```python
from build123d import *

# Parameters (mm, degrees)
BOSS_EXTRUDE1_DEPTH = 4.5
CUT_EXTRUDE1_DEPTH  = 24.873773295
FILLET1_R           = 10
FILLET2_R           = 1


with BuildPart() as part:
    # Sketch1 → Boss-Extrude1 (new body)
    with BuildSketch(Plane.XY):
        with BuildLine():
            ThreePointArc((1.715540677, -1.028066236), (0, 2), (-1.715540677, -1.028066236))
            ThreePointArc((-1.715540677, -1.028066236), (-12.4000088, -2.631992998), (-22.452233946, -6.592196245))
            ThreePointArc((-22.452233946, -6.592196245), (-18.208029962, 2.594911639), (-8.117877526, 3.372756458))
            ThreePointArc((-8.117877526, 3.372756458), (0, 4), (8.117877526, 3.372756458))
            ThreePointArc((8.117877526, 3.372756458), (18.208029962, 2.594911639), (22.452233946, -6.592196245))
            ThreePointArc((22.452233946, -6.592196245), (12.4000088, -2.631992998), (1.715540677, -1.028066236))
        make_face()
    extrude(amount=BOSS_EXTRUDE1_DEPTH)

    # Sketch2 → Cut-Extrude1 (cut, through all)
    with BuildSketch(Plane.XY.offset(4.5)):
        with BuildLine():
            ThreePointArc((-3.908816698, 0.849206701), (0, -98.692698318), (3.908816698, 0.849206701))
            ThreePointArc((3.908816698, 0.849206701), (0, -4), (-3.908816698, 0.849206701))
        make_face()
    extrude(amount=-CUT_EXTRUDE1_DEPTH, mode=Mode.SUBTRACT)

    # Fillet1
    # the kernel refuses this fillet: 10 mm, written as the material it adds along each edge
    with BuildSketch(Plane(origin=(3.908816698, 0.849206701, 4.5), x_dir=(0.9890559129703541, -0.14754118414320608, 0), z_dir=(0, 0, -1))) as fillet1_piece_1:
        with BuildLine():
            CenterArc((6.236508998, 9.975798703), FILLET1_R, 232.997328349, 40.989656439)
            Line((0.217986376, 1.989724232), (0.097615924, 1.830002743))
            ThreePointArc((0.097615924, 1.830002743), (0.036653136, 1.002787408), (-0.187037265, 0.070831218))
            Line((-0.187037265, 0.070831218), (-0.013905973, -0.199515974))
            ThreePointArc((-0.013905973, -0.199515974), (3.465903834, -0.320637896), (6.945713641, -0.199515974))
            Line((6.945713641, -0.199515974), (6.931807668, 0))
        make_face()
    extrude(amount=4.5)
    with BuildSketch(Plane(origin=(-3.908816698, 0.849206701, 4.5), x_dir=(-0.9890559129703533, -0.14754118414321077, 0), z_dir=(0, 0, -1))) as fillet1_piece_2:
        with BuildLine():
            CenterArc((6.236508998, -9.975798703), FILLET1_R, 86.013015212, 40.989656439)
            Line((0.217986376, -1.989724232), (0.097615924, -1.830002743))
            ThreePointArc((0.097615924, -1.830002743), (0.036653136, -1.002787408), (-0.187037265, -0.070831218))
            Line((-0.187037265, -0.070831218), (-0.013905973, 0.199515974))
            ThreePointArc((-0.013905973, 0.199515974), (3.465903834, 0.320637896), (6.945713641, 0.199515974))
            Line((6.945713641, 0.199515974), (6.931807668, 0))
        make_face()
    extrude(amount=4.5)

    # Fillet2
    fillet2_edges = [part.edges().sort_by_distance(p)[0] for p in [
        (-8.117877526, 3.372756458, 2.25),
        (8.117877526, 3.372756458, 2.25),
        (22.415896296, -4.321740675, 2.25),
        (-22.415896296, -4.321740675, 2.25),
    ]]
    fillet(fillet2_edges, radius=FILLET2_R)


solid = part.part
```
Geometry: final body of the model. Coordinates: model frame, mm. A direction names the side the tool comes from. Coordinates: 2 decimals unless noted, no trailing zeros. Order: outer loops, then holes, each group sorted by start corner. A loop starts at its lowest first (then second) coordinate and runs counter-clockwise, first axis right, second up. Notation, with made-up numbers: M 50.25,-16 L 100.25,-16 A25 ccw 100.25,-1 Z; hole C 66,57 d9. An arc over 180 degrees is marked long. Answer as CSV lines item,"result".
Q1. Line query: probe 1 along X at (y, z) = (0.25, 2); probe 2 along Y at (x, z) = (18.5, 2.5); probe 3 along X at (y, z) = (0.5, 0.85). Output: solid intervals per line, ascending. Write a range as [from, to].
Answers:
probe 1,"x = [-20.6, -1.98], [1.98, 20.6]"
probe 2,"y = [-2.56, 2.38]"
probe 3,"x = [-20.41, -1.94], [1.94, 20.41]"
Q2. Section B-B on x = 0. Return the cut outline in (y, z).
Answers:
outline,"M 2,0 L 4,0 L 4,4.5 L 2,4.5 Z"
Q3. Section A-A on y = 1. Return the cut outline in (x, z), and give its area (3 significant figures).
Answers:
outline,"M -20,0 L -1.73,0 L -1.73,4.5 L -20,4.5 Z; M 1.73,0 L 20,0 L 20,4.5 L 1.73,4.5 Z"
area,"164 mm^2"
Q4. Set-up query: faces 1 (the cylindrical face through (0, 2, 2)), 2 (the cylindrical face through (-15.666, -1.523, 2.281)). Return all of +Z, -Z, +X, -X, +Y, -Y with unobstructed straight access to the full face (end or side cutting, diameter ignored); none if empty.
Answers:
face 1,"+Z, -Z"
face 2,"+Z, -Z, -Y"
Q5. Draft query along X for faces 3 (the cylindrical face through (7.16, -0.043, 2.282)), 4 (the flat face through (-1, 3, 4.5)). Return one class per face: pulls with the +X half, pulls with the -X half, needs draft (parallel to the pull), parting line crosses it, or undercut.
Answers:
face 3,"undercut"
face 4,"needs draft"
Q6. Section C-C on x = 19. Return the cut outline in (y, z), and give its area (3 significant figures).
Answers:
outline,"M -2.76,0 L 1.98,0 L 1.98,4.5 L -2.76,4.5 Z"
area,"21.3 mm^2"
Q7. First-contact query: P1, Ø2, axis at x = -10, z = 3.5, coming from the +Y side; P2, Ø1.5, axis at x = 9, z = 3, coming from the -Y side; P3, Ø1, axis at x = 13, z = 1.5, coming from the -Y side. Flat tips, straight axial feed; report the tip coordinate or a pass-through.
Answers:
P1,"stops at y = 4.27"
P2,"stops at y = 0"
P3,"stops at y = -0.86"
